Input: part model. Units: mm. Frame: model coordinates. Face numbers are marked on the shaded views. A direction names the side the tool comes from. Give positions to 0.01 mm unless a question says otherwise; leave off trailing zeros. Order: outer loops, then holes, each group sorted by start corner. A loop starts at its lowest first (then second) coordinate and runs counter-clockwise, first axis right, second up. Notation, with made-up numbers: M 13.25,61.25 L 58.25,61.25 A13 cw 58.25,65.25 Z; hole C -3.75,-26 d10. An arc over 180 degrees is marked long. Use a Markdown table: item, result.
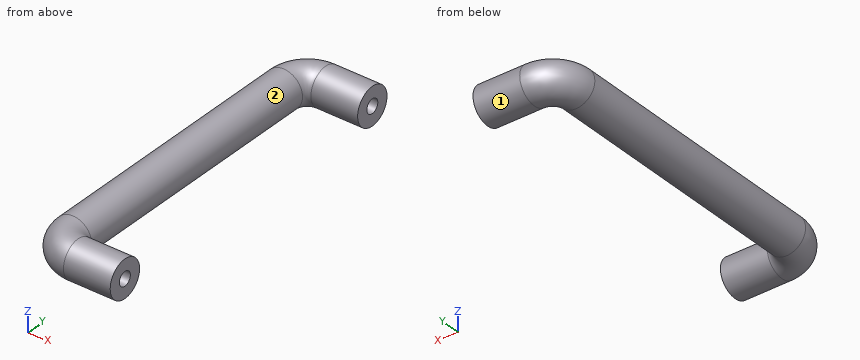
Autodesk Inventor part; units mm, degrees
ref_plane "YZ Plane" through (0, 0, 0) normal (1, 0, 0) x (0, 1, 0)
ref_plane "XZ Plane" through (0, 0, 0) normal (0, 1, 0) x (-1, 0, 0)
ref_plane "XY Plane" through (0, 0, 0) normal (0, 0, 1) x (1, 0, 0)
sketch "Sketch3" plane through (0, 0, 0) normal (1, 0, 0) x (0, 1, 0)
  circle A0 centre (0, 0) radius 8
  circle A1 centre (0, 0) radius 3
  dimension "d4" = 16
  dimension "d5" = 6
sketch "Sketch4" plane through (0, 0, 0) normal (0, 0, 1) x (1, 0, 0)
  line L0 (0, 0) -> (-20, 0)
  line L1 (-30, -10) -> (-30, -96)
  arc A0 (-20, 0) -> (-30, -10) centre (-20, -10) ccw
  line L2 (0, -134.8) -> (-20, -134.8)
  line L3 (-20, -134.8) -> (-20, -134.8)
  line L4 (-30, -124.8) -> (-30, -96)
  arc A1 (-30, -124.8) -> (-20, -134.8) centre (-20, -124.8) ccw
  point P0 (-30, -106)
  point P1 (-30, -134.8)
sweep "Sweep2" add profiles "Sketch3" path "Sketch4"
equation "\"BendRadius\" = Thickness"
equation "\"BendReliefWidth\" = Thickness"
equation "\"BendReliefDepth\" = 0.5 * Thickness"
equation "\"CornerReliefSize\" = 4 * Thickness"
equation "\"MinimumRemnant\" = 2 * Thickness"
equation "\"TransitionRadius\" = BendRadius"
equation "\"JacobiRadiusSize\" = BendRadius"
equation "\"GapSize\" = Thickness"
properties part number "Rubber pipe turn"
1) Cut plane D-D on z = -6.5. Return loops of the section in (x, y), and give its area (3 significant figures).
Response values:
| item | result |
|---|---|
| outline | M -34.66,-124.8 A14.66 ccw -20,-139.46 L 0,-139.46 L 0,-130.14 L -20,-130.14 A5.34 cw -25.34,-124.8 L -25.34,-10 A5.34 cw -20,-4.66 L 0,-4.66 L 0,4.66 L -20,4.66 A14.66 ccw -34.66,-10 Z |
| area | 1,740 mm² |
2) Cut plane B-B on z = 0. Return loops of the section in (x, y), and give its area (3 significant figures).
Response values:
| item | result |
|---|---|
| outline | M -38,-124.8 A18 ccw -20,-142.8 L 0,-142.8 L 0,-137.8 L -20,-137.8 A13 cw -33,-124.8 L -33,-10 A13 cw -20,3 L 0,3 L 0,8 L -20,8 A18 ccw -38,-10 Z; M -27,-124.8 A7 ccw -20,-131.8 L 0,-131.8 L 0,-126.8 L -20,-126.8 A2 cw -22,-124.8 L -22,-10 A2 cw -20,-8 L 0,-8 L 0,-3 L -20,-3 A7 ccw -27,-10 Z |
| area | 1,860 mm² |
3) Cut plane C-C on y = -46. Return loops of the section in (x, z), and give its area (3 significant figures).
Response values:
| item | result |
|---|---|
| outline | C -30,0 d16; hole C -30,0 d6 |
| area | 173 mm² |
4) Cut plane A-A on x = -4.5. Return loops of the section in (y, z), and give its area (3 significant figures).
Response values:
| item | result |
|---|---|
| outline | C -134.8,0 d16; C 0,0 d16; hole C -134.8,0 d6; hole C 0,0 d6 |
| area | 346 mm² |
5) Reachability of the marked faces 1 and 2 from +Z, -Z, +X, -X, +Y, -Y: full face, straight path, thin tool, end or side. Return the list, or none.
Response values:
| item | result |
|---|---|
| face 1 | +X |
| face 2 | none |
6) First-contact query: pin 1 Ø3.5 at (x, z) = (-30, 0) entering from -Y; pin 2 Ø7 at (y, z) = (-134.8, 0) entering from -X; pin 3 Ø6 at (x, z) = (-13, -4.5) entering from +Y. Flat tips, straight axial feed; report the tip coordinate or a pass-through.
Response values:
| item | result |
|---|---|
| pin 1 | stops at y = -140.8 |
| pin 2 | stops at x = -36.79 |
| pin 3 | stops at y = 7.86 |
7) Material intervals for line 1 (Y direction, x = -11.25, z = 0); line 2 (X direction, y = -48, z = 0); line 3 (Y direction, x = -23.5, z = 1), sorted ascending. Write a range as from..to.
Response values:
| item | result |
|---|---|
| line 1 | y = -142.8..-137.8, -131.8..-126.8, -8..-3, 3..8 |
| line 2 | x = -38..-33, -27..-22 |
| line 3 | y = -142.39..-137.14, -131.06..-3.74, 2.34..7.59 |
